from build123d import *

# Parameters (mm, degrees)
SKETCH1_R             = 1.25
BOSS_EXTRUDE1_DEPTH   = 3
BOSS_EXTRUDE1_2_DEPTH = 3
BOSS_EXTRUDE2_DEPTH   = 14
FILLET1_R             = 1


with BuildPart() as part:
    # Sketch1 → Boss-Extrude1 (new body)
    with BuildSketch(Plane.XY):
        with BuildLine():
            Line((0, -7), (60, -7))
            Line((60, -7), (60, -4))
            add(Edge.make_bspline(
                [(60, -4), (55.163320485, -4), (49.053298786, -3.947636788), (42.55073288, -3.579164898)],
                knots=[0, 0, 0, 0, 0.318433517, 0.318433517, 0.318433517, 0.318433517], degree=3))
            ThreePointArc((42.55073288, -3.579164898), (40.208782774, 0.992726141), (37.254706676, -3.209696062))
            add(Edge.make_bspline(
                [(37.254706676, -3.209696062), (24.804076794, -2.167051335), (11.80488785, 0.231594042), (4.038655229, 5.717452574)],
                knots=[0.403779051, 0.403779051, 0.403779051, 0.403779051, 1, 1, 1, 1], degree=3))
            ThreePointArc((4.038655229, 5.717452574), (6.671662762, -2.118706207), (0, -7))
        make_face()
        with Locations((40, -2)):
            Circle(SKETCH1_R, mode=Mode.SUBTRACT)
    extrude(amount=BOSS_EXTRUDE1_DEPTH)



with BuildPart() as body_2:
    # Sketch1 → Boss-Extrude1 2 (new body)
    with BuildSketch(Plane.XY):
        with BuildLine():
            Line((-60, -7), (0, -7))
            ThreePointArc((0, -7), (-6.671662763, -2.118706204), (-4.038655225, 5.717452578))
            add(Edge.make_bspline(
                [(-4.038655225, 5.717452578), (-11.80488784, 0.231594059), (-24.804076837, -2.16705132), (-37.254706671, -3.209696052)],
                knots=[0.403779054, 0.403779054, 0.403779054, 0.403779054, 1, 1, 1, 1], degree=3))
            ThreePointArc((-37.254706671, -3.209696052), (-40.208782776, 0.992726141), (-42.550732884, -3.579164892))
            add(Edge.make_bspline(
                [(-42.550732884, -3.579164892), (-49.053298864, -3.94763679), (-55.163320586, -4), (-60, -4)],
                knots=[1.085345534, 1.085345534, 1.085345534, 1.085345534, 1.403779054, 1.403779054, 1.403779054, 1.403779054], degree=3))
            Line((-60, -4), (-60, -7))
        make_face()
        with Locations((-40, -2)):
            Circle(SKETCH1_R, mode=Mode.SUBTRACT)
    extrude(amount=BOSS_EXTRUDE1_2_DEPTH)


with BuildPart() as part_1:
    add(part.part)

    add(body_2.part)  # Boss-Extrude2 merges body 2
    # Sketch1_3 → Boss-Extrude2 (add)
    with BuildSketch(Plane.XY):
        with BuildLine():
            ThreePointArc((-5.744562647, -4), (-3.240370349, -6.204836823), (0, -7))
            Line((0, -7), (0, -4.15))
            ThreePointArc((0, -4.15), (-0.55789784, -4.112329024), (-1.105667219, -4))
            Line((-1.105667219, -4), (-5.744562647, -4))
        make_face()
        with BuildLine():
            Line((0, -4.15), (0, -7))
            ThreePointArc((0, -7), (3.240370349, -6.204836823), (5.744562647, -4))
            Line((5.744562647, -4), (1.105667219, -4))
            ThreePointArc((1.105667219, -4), (0.55789784, -4.112329024), (0, -4.15))
        make_face()
        with BuildLine():
            ThreePointArc((-4.038655225, 5.717452578), (-6.894567363, 1.210347418), (-5.744562647, -4))
            Line((-5.744562647, -4), (-1.105667219, -4))
            ThreePointArc((-1.105667219, -4), (-4.112329024, 0.55789784), (0, 4.15))
            Line((0, 4.15), (0, 7))
            ThreePointArc((0, 7), (-2.118706204, 6.671662763), (-4.038655225, 5.717452578))
        make_face()
        with BuildLine():
            Line((1.105667219, -4), (5.744562647, -4))
            ThreePointArc((5.744562647, -4), (6.678770041, -2.096194346), (7, 0))
            ThreePointArc((7, 0), (6.215729507, 3.219426455), (4.038655229, 5.717452574))
            ThreePointArc((4.038655229, 5.717452574), (2.118706207, 6.671662762), (0, 7))
            Line((0, 7), (0, 4.15))
            ThreePointArc((0, 4.15), (2.934493142, 2.934493142), (4.15, 0))
            ThreePointArc((4.15, 0), (3.302349085, -2.513362393), (1.105667219, -4))
        make_face()
    extrude(amount=BOSS_EXTRUDE2_DEPTH)

    # Fillet1
    fillet1_edges = [part_1.edges().sort_by_distance(p)[0] for p in [
        (38.75, -2, 3),
        (38.75, -2, 0),
        (-41.25, -2, 3),
        (-41.25, -2, 0),
    ]]
    fillet(fillet1_edges, radius=FILLET1_R)


solid = part_1.part
Read the model definition and answer for the solid it produces. Units are mm, in the model's axes. Round coordinates to 2 decimals unless told otherwise and drop trailing zeros. Write each loop counter-clockwise with the first axis right and the second up, starting at its lowest first coordinate (ties: lowest second). Pieces come first, ordered by that corner, then holes.
1. Determine the mould class of faces 1 (the face through (38.75, -1.95, 1.49)), 2 (the face through (-41.25, -1.95, 1.49)), 3 (the face through (-60, -5, 1)), 4 (the face through (25, -4, 3)) for opening direction X: pulls with the +X half, pulls with the -X half, needs draft (parallel to the pull), parting line crosses it, or undercut.
2. Straight lines are drawn through the part: L1, parallel to Y at x = -40, z = 1.85; L2, parallel to Z at x = 6, y = 4; L3, parallel to X at y = 2.25, z = 8.75. For each, find the intervals that lie inside material, in ascending order.
3. The part is cut by section B-B, the plane z = 10.5. Determine the outline of the cut face in (x, y), then the cut area to 3 significant figures.
4. Given pin 1 Ø4 at (x, y) = (39, -3) entering from +Z; pin 2 Ø1 at (y, z) = (-5, 4.5) entering from -X; pin 3 Ø3 at (y, z) = (5, 3) entering from -X, each flat-ended and moving along its own axis, determine where each tip first touches the part or whether it passes through.
5. The part is cut by section C-C, the plane y = -2. State how many separate pieces and enclosed holes the cut face has, then the cut area to 3 significant figures.
6. The part is cut by section A-A, the plane x = 40. Determine the outline of the cut face in (y, z).
Values:
1. face 1: undercut
1. face 2: undercut
1. face 3: pulls with the -X half
1. face 4: needs draft
2. L1: y = -7 to -3.25, -0.75 to 1
2. L2: z = 0 to 3
2. L3: x = -6.63 to -3.49, 3.49 to 6.63
3. outline: circle Ø14 at (0, 0); hole circle Ø8.3 at (0, 0)
3. area: 99.8 mm2
4. pin 1: stops at z = 3
4. pin 2: stops at x = -5.36
4. pin 3: stops at x = -7.77
5. separate pieces: 6
5. enclosed holes: 0
5. area: 227 mm2
6. outline: (-7, 0) - (-4.25, 0) arc R1 ccw to (-3.25, 1) - (-3.25, 2) arc R1 ccw to (-4.25, 3) - (-7, 3) - close; (-0.75, 1) arc R1 ccw to (0.25, 0) - (1, 0) - (1, 3) - (0.25, 3) arc R1 ccw to (-0.75, 2) - close
